For this review, take the finished solid that the model builds, in its own axes (mm). A direction names the side the tool comes from. Round coordinates to 2 decimals unless told otherwise and drop trailing zeros. Loops run counter-clockwise (first coordinate to the right, second up) from the corner with the lowest first, then second, coordinate; pieces in that order, holes last.
1. Consider section C-C on x = -78.5. State the section outline as (y, z) points (3 decimals), then the cut area to 3 significant figures.
2. Tool access review of faces 1 (the cylindrical face through (77.98, -72.54, 5.94)), 2 (the flat face through (117.5, -1, 36)): name each direction out of +Z, -Z, +X, -X, +Y, -Y from which nothing blocks a thin tool from reaching the whole face with its end or side.
3. To check wall thickness, follow line 1 along Y through (x, z) = (-78.5, 9) (3 decimals); line 2 along Y through (x, z) = (95, 24); line 3 along X through (y, z) = (-51, 61.5). State the ranges of each line that lie inside material, in increasing order.
4. Clearance check with flat-ended pins moving along their axes: pin 1 Ø4 at (x, y) = (80.5, -78.5) entering from +Z; pin 2 Ø3 at (x, z) = (-111.5, 24.5) entering from -Y; pin 3 Ø4 at (y, z) = (-90, 35) entering from +X; pin 4 Ø5.5 at (x, y) = (113, 53) entering from +Z. State where each tip first meets the part, or that it passes through.
5. Consider section A-A on x = 6. State the section outline as (y, z) points, then the cut area to 3 significant figures.
6. Draft analysis for pull direction Y (two halves, no side actions). For faces 3 (the flat face through (110.5, 42, 4)), 4 (the cylindrical face through (115.094, 92.719, 37.518)), 5 (the cylindrical face through (115.094, -92.719, 37.518)), state which applies: released by +Y, released by -Y, zero draft, split by the parting line, or undercut.
7. Consider section B-B on y = -34.5. State the section outline as (x, z) points, then the cut area to 3 significant figures.
from build123d import *

# Parameters (mm, degrees)
SKETCH1_W           = 235
SKETCH1_H           = 190
BOSS_EXTRUDE1_DEPTH = 74
CUT_EXTRUDE1_DEPTH  = 72
FILLET1_R           = 2
FILLET2_R           = 5
SKETCH3_R           = 4
BOSS_EXTRUDE2_DEPTH = 8
FILLET3_R           = 8
SKETCH4_R           = 3
CUT_EXTRUDE2_DEPTH  = 3
SKETCH5_W           = 1
SKETCH5_H           = 165
BOSS_EXTRUDE3_DEPTH = 5
SKETCH6_W           = 115.5
SKETCH6_H           = 1.5
BOSS_EXTRUDE4_DEPTH = 5
BOSS_EXTRUDE5_DEPTH = 1.5
SKETCH8_W           = 5
SKETCH8_H           = 2.5
CUT_EXTRUDE3_DEPTH  = 5


with BuildPart() as part:
    # Sketch1 → Boss-Extrude1 (new body)
    with BuildSketch(Plane.XY):
        Rectangle(SKETCH1_W, SKETCH1_H)
    extrude(amount=BOSS_EXTRUDE1_DEPTH)

    # Sketch2 → Cut-Extrude1 (cut)
    with BuildSketch(Plane.XY.offset(74)):
        Polygon((105, 93), (-105, 93), (-105, 82.5), (-115.5, 82.5), (-115.5, -82.5), (-105, -82.5), (-105, -93), (105.534797486, -93), (105.534797486, -82.5), (115.5, -82.5), (115.5, 82.5), (105, 82.5), align=None)
    extrude(amount=-CUT_EXTRUDE1_DEPTH, mode=Mode.SUBTRACT)

    # Fillet1
    fillet1_edges = [part.edges().sort_by_distance(p)[0] for p in [
        (-105, -93, 38),
        (-115.5, -82.5, 38),
        (-115.5, 82.5, 38),
        (-105, 93, 38),
        (105, 93, 38),
        (115.5, 82.5, 38),
        (115.5, -82.5, 38),
        (105.534797486, -93, 38),
    ]]
    fillet(fillet1_edges, radius=FILLET1_R)

    # Fillet2
    fillet2_edges = [part.edges().sort_by_distance(p)[0] for p in [
        (-105, -82.5, 38),
        (-105, 82.5, 38),
        (105, 82.5, 38),
        (105.534797486, -82.5, 38),
    ]]
    fillet(fillet2_edges, radius=FILLET2_R)

    # Sketch3 → Boss-Extrude2 (add)
    with BuildSketch(Plane.XY.offset(2)):
        with Locations((-78.5, 76.505)):
            Circle(SKETCH3_R)
        with Locations((78.5, 76.505)):
            Circle(SKETCH3_R)
        with Locations((78.5, -76.505)):
            Circle(SKETCH3_R)
        with Locations((-78.5, -76.505)):
            Circle(SKETCH3_R)
    extrude(amount=BOSS_EXTRUDE2_DEPTH)

    # Fillet3
    fillet3_edges = [part.edges().sort_by_distance(p)[0] for p in [
        (117.5, -95, 37),
        (-117.5, -95, 37),
        (-117.5, 95, 37),
        (117.5, 95, 37),
    ]]
    fillet(fillet3_edges, radius=FILLET3_R)

    # Sketch4 → Cut-Extrude2 (cut)
    with BuildSketch(Plane.XY.offset(10)):
        with Locations((78.5, 76.505)):
            Circle(SKETCH4_R)
        with Locations((78.5, -76.505)):
            Circle(SKETCH4_R)
        with Locations((-78.5, -76.505)):
            Circle(SKETCH4_R)
        with Locations((-78.5, 76.505)):
            Circle(SKETCH4_R)
    extrude(amount=-CUT_EXTRUDE2_DEPTH, mode=Mode.SUBTRACT)

    # Sketch5 → Boss-Extrude3 (add)
    with BuildSketch(Plane.XY.offset(2)):
        with Locations((110, 0)):
            Rectangle(SKETCH5_W, SKETCH5_H)
    extrude(amount=BOSS_EXTRUDE3_DEPTH)

    # Sketch6 → Boss-Extrude4 (add)
    with BuildSketch(Plane.XY.offset(2)):
        with Locations((57.75, 2)):
            Rectangle(SKETCH6_W, SKETCH6_H)
        with Locations((57.75, -2)):
            Rectangle(SKETCH6_W, SKETCH6_H)
    extrude(amount=BOSS_EXTRUDE4_DEPTH)

    # Sketch7 → Boss-Extrude5 (add)
    with BuildSketch(Plane.XZ.offset(2.75)):
        Polygon((107.5, 7), (115.5, 64), (115.5, 7), align=None)
    boss_extrude5 = extrude(amount=-BOSS_EXTRUDE5_DEPTH)

    # Mirror1: Boss-Extrude5 across plane
    add(boss_extrude5.mirror(Plane.ZX))

    # Sketch8 → Cut-Extrude3 (cut)
    with BuildSketch(Plane.ZY.offset(-109.5)):
        with Locations((4.5, 0)):
            Rectangle(SKETCH8_W, SKETCH8_H)
    extrude(amount=-CUT_EXTRUDE3_DEPTH, mode=Mode.SUBTRACT)


solid = part.part
Resolved:
1. outline: (-95, 0) - (95, 0) - (95, 74) - (93, 74) - (93, 2) - (80.505, 2) - (80.505, 10) - (79.505, 10) - (79.505, 7) - (73.505, 7) - (73.505, 10) - (72.505, 10) - (72.505, 2) - (-72.505, 2) - (-72.505, 10) - (-73.505, 10) - (-73.505, 7) - (-79.505, 7) - (-79.505, 10) - (-80.505, 10) - (-80.505, 2) - (-93, 2) - (-93, 74) - (-95, 74) - close
1. area: 760 mm2
2. face 1: +Z
2. face 2: +Z, -Z, +X, +Y, -Y
3. line 1: y = -95 to -93, -80.505 to -79.505, -73.505 to -72.505, 72.505 to 73.505, 79.505 to 80.505, 93 to 95
3. line 2: y = -95 to -93, 93 to 95
3. line 3: x = -117.5 to -115.5, 115.5 to 117.5
4. pin 1: stops at z = 10
4. pin 2: stops at y = -94.98
4. pin 3: stops at x = 117.44
4. pin 4: stops at z = 74
5. outline: (-95, 0) - (95, 0) - (95, 74) - (93, 74) - (93, 2) - (2.75, 2) - (2.75, 7) - (1.25, 7) - (1.25, 2) - (-1.25, 2) - (-1.25, 7) - (-2.75, 7) - (-2.75, 2) - (-93, 2) - (-93, 74) - (-95, 74) - close
5. area: 683 mm2
6. face 3: undercut
6. face 4: released by +Y
6. face 5: released by -Y
7. outline: (-117.5, 0) - (117.5, 0) - (117.5, 74) - (115.5, 74) - (115.5, 2) - (110.5, 2) - (110.5, 7) - (109.5, 7) - (109.5, 2) - (-115.5, 2) - (-115.5, 74) - (-117.5, 74) - close
7. area: 763 mm2
